Source: CAD feature listing. Evaluate the final solid. Frame: model axes, mm. Round coordinates to 2 decimals unless told otherwise and drop trailing zeros. Loops run counter-clockwise (first coordinate to the right, second up) from the corner with the lowest first, then second, coordinate; pieces in that order, holes last. Notation, with made-up numbers: M 41,-26.5 L 85,-26.5 A5 cw 85,-17.5 Z; hole C 83,59 d3. An arc over 180 degrees is marked long. One line per item, written item: value.
from build123d import *

# Parameters (mm, degrees)
SZKIC1_R                    = 1.7
SZKIC1_R_2                  = 2.15
DODANIE_WYCI_GNI_CIE1_DEPTH = 5


with BuildPart() as part:
    # Szkic1 → Dodanie-wyciągnięcie1 (new body)
    with BuildSketch(Plane.XY):
        with BuildLine():
            Line((0, -12), (-54.784750049, -12))
            ThreePointArc((-54.784750049, -12), (-66.784750049, 0), (-54.784750049, 12))
            Line((-54.784750049, 12), (0, 12))
            ThreePointArc((0, 12), (12, 0), (0, -12))
        make_face()
        with Locations((0, 7.001028496)):
            Circle(SZKIC1_R, mode=Mode.SUBTRACT)
        Circle(SZKIC1_R_2, mode=Mode.SUBTRACT)
        with Locations((7.001028496, 0)):
            Circle(SZKIC1_R, mode=Mode.SUBTRACT)
        with Locations((0, -7.001028496)):
            Circle(SZKIC1_R, mode=Mode.SUBTRACT)
        with Locations((-7.001028496, 0)):
            Circle(SZKIC1_R, mode=Mode.SUBTRACT)
        with Locations(Location((-47.783721554, 0, 0), (0, 0, 180))):
            Circle(SZKIC1_R, mode=Mode.SUBTRACT)
        with Locations(Location((-54.784750049, -7.001028496, 0), (0, 0, 180))):
            Circle(SZKIC1_R, mode=Mode.SUBTRACT)
        with Locations(Location((-61.785778545, 0, 0), (0, 0, 180))):
            Circle(SZKIC1_R, mode=Mode.SUBTRACT)
        with Locations(Location((-54.784750049, 0, 0), (0, 0, 180))):
            Circle(SZKIC1_R_2, mode=Mode.SUBTRACT)
        with Locations(Location((-54.784750049, 7.001028496, 0), (0, 0, 180))):
            Circle(SZKIC1_R, mode=Mode.SUBTRACT)
    extrude(amount=DODANIE_WYCI_GNI_CIE1_DEPTH)


solid = part.part
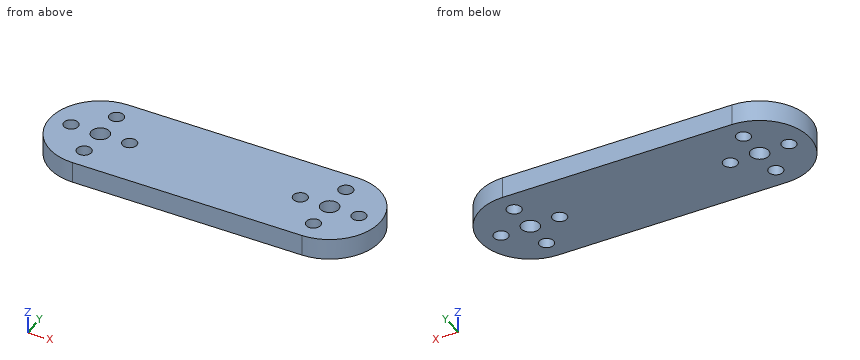
1. Section query B-B (x = 6.5). Return the cut outline in (y, z), and give its area (3 significant figures).
Report:
outline: M -10.09,0 L -1.62,0 L -1.62,5 L -10.09,5 Z; M 1.62,0 L 10.09,0 L 10.09,5 L 1.62,5 Z
area: 84.6 mm2
2. Section query C-C (z = 3.85). Count the separate pieces of the cut face and the enclosed holes in it, and give its area (3 significant figures).
Report:
separate pieces: 1
enclosed holes: 10
area: 1,670 mm2
3. Ray query, line 1 (Y direction, x = 0, z = 1.15); line 2 (X direction, y = -6.75, z = 2.25); line 3 (X direction, y = -5.5, z = 4.2). Return the intervals inside material, ascending. Write a range as [from, to].
Report:
line 1: y = [-12, -8.7], [-5.3, -2.15], [2.15, 5.3], [8.7, 12]
line 2: x = [-64.71, -56.47], [-53.1, -1.68], [1.68, 9.92]
line 3: x = [-65.45, -55.58], [-53.99, -0.8], [0.8, 10.67]
4. Section query A-A (y = 0). Return the cut outline in (x, z), and give its area (3 significant figures).
Report:
outline: M -66.78,0 L -63.49,0 L -63.49,5 L -66.78,5 Z; M -60.09,0 L -56.93,0 L -56.93,5 L -60.09,5 Z; M -52.63,0 L -49.48,0 L -49.48,5 L -52.63,5 Z; M -46.08,0 L -8.7,0 L -8.7,5 L -46.08,5 Z; M -5.3,0 L -2.15,0 L -2.15,5 L -5.3,5 Z; M 2.15,0 L 5.3,0 L 5.3,5 L 2.15,5 Z; M 8.7,0 L 12,0 L 12,5 L 8.7,5 Z
area: 283 mm2
5. Pin query (flat end, axial travel): pin 1 (3 mm diameter, centred on x = 0, y = -7, fed in from -Z); pin 2 (1.5 mm diameter, centred on y = 9.5, z = 4, fed in from +X). Return the tip coordinate at first contact, or that it passes through.
Report:
pin 1: passes through
pin 2: stops at x = 8.21
